Model file for the job. Use its own axes, mm. Round coordinates to 2 decimals unless told otherwise and drop trailing zeros. Order: outer loops, then holes, each group sorted by start corner. A loop starts at its lowest first (then second) coordinate and runs counter-clockwise, first axis right, second up. Notation, with made-up numbers: (64.5, 5.5) -> (79.5, 5.5) arc R15 cw to (79.5, 31.5) -> close; hole circle Ø5 at (-38, 57.5). An arc over 180 degrees is marked (long way). Answer as CSV lines item,"result".
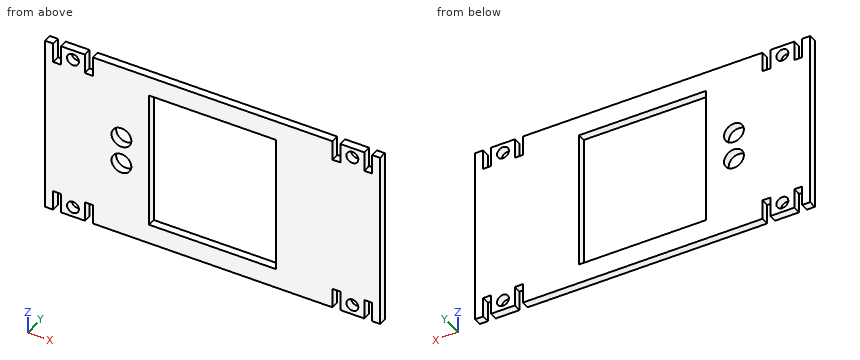
```python
from build123d import *

# Parameters (mm, degrees)
SKETCH1_R           = 1.5
BOSS_EXTRUDE1_DEPTH = 2
SKETCH2_W           = 32
SKETCH2_H           = 35
CUT_EXTRUDE1_DEPTH  = 10
SKETCH3_R           = 2.5
CUT_EXTRUDE2_DEPTH  = 10


with BuildPart() as part:
    # Sketch1 → Boss-Extrude1 (new body)
    with BuildSketch(Plane(origin=(0, 0, 0), x_dir=(1, 0, 0), z_dir=(0, 1, 0))):
        Polygon((0, 0), (2, 0), (2, 5), (4, 5), (4, 0), (10, 0), (10, 5), (12, 5), (12, 0), (72.4, 0), (72.4, 5), (74.4, 5), (74.4, 0), (80.4, 0), (80.4, 5), (82.4, 5), (82.4, 0), (84.4, 0), (84.4, 45), (82.4, 45), (82.4, 40), (80.4, 40), (80.4, 45), (74.4, 45), (74.4, 40), (72.4, 40), (72.4, 45), (12, 45), (12, 40), (10, 40), (10, 45), (4, 45), (4, 40), (2, 40), (2, 45), (0, 45), align=None)
        with Locations(Location((7, 42.5, 0), (0, 0, 270))):
            Circle(SKETCH1_R, mode=Mode.SUBTRACT)
        with Locations(Location((77.4, 42.5, 0), (0, 0, 90))):
            Circle(SKETCH1_R, mode=Mode.SUBTRACT)
        with Locations(Location((7, 2.5, 0), (0, 0, 90))):
            Circle(SKETCH1_R, mode=Mode.SUBTRACT)
        with Locations(Location((77.4, 2.5, 0), (0, 0, 270))):
            Circle(SKETCH1_R, mode=Mode.SUBTRACT)
    extrude(amount=BOSS_EXTRUDE1_DEPTH)

    # Sketch2 → Cut-Extrude1 (cut)
    with BuildSketch(Plane(origin=(0, 2, 0), x_dir=(1, 0, 0), z_dir=(0, 1, 0))):
        with Locations((42.2, 22.5)):
            Rectangle(SKETCH2_W, SKETCH2_H)
    extrude(amount=-CUT_EXTRUDE1_DEPTH, mode=Mode.SUBTRACT)

    # Sketch3 → Cut-Extrude2 (cut)
    with BuildSketch(Plane(origin=(0, 2, 0), x_dir=(1, 0, 0), z_dir=(0, 1, 0))):
        with Locations(Location((19.2, 26, 0), (0, 0, 270))):
            Circle(SKETCH3_R)
        with Locations(Location((19.2, 19, 0), (0, 0, 90))):
            Circle(SKETCH3_R)
    extrude(amount=-CUT_EXTRUDE2_DEPTH, mode=Mode.SUBTRACT)


solid = part.part
```
Q1. Saw through at C-C (x = 36). Write the cut outline in (y, z).
Checks:
outline,"(0, -45) -> (2, -45) -> (2, -40) -> (0, -40) -> close; (0, -5) -> (2, -5) -> (2, 0) -> (0, 0) -> close"
Q2. Saw through at B-B (z = -32). Write the cut outline in (x, y), plus the area to 3 significant figures.
Checks:
outline,"(0, 0) -> (26.2, 0) -> (26.2, 2) -> (0, 2) -> close; (58.2, 0) -> (84.4, 0) -> (84.4, 2) -> (58.2, 2) -> close"
area,"105 mm²"
Q3. Saw through at D-D (z = -2.5). Write the cut outline in (x, y).
Checks:
outline,"(0, 0) -> (2, 0) -> (2, 2) -> (0, 2) -> close; (4, 0) -> (5.5, 0) -> (5.5, 2) -> (4, 2) -> close; (8.5, 0) -> (10, 0) -> (10, 2) -> (8.5, 2) -> close; (12, 0) -> (72.4, 0) -> (72.4, 2) -> (12, 2) -> close; (74.4, 0) -> (75.9, 0) -> (75.9, 2) -> (74.4, 2) -> close; (78.9, 0) -> (80.4, 0) -> (80.4, 2) -> (78.9, 2) -> close; (82.4, 0) -> (84.4, 0) -> (84.4, 2) -> (82.4, 2) -> close"
Q4. Saw through at A-A (x = 19.2). Write the cut outline in (y, z).
Checks:
outline,"(0, -45) -> (2, -45) -> (2, -28.5) -> (0, -28.5) -> close; (0, -23.5) -> (2, -23.5) -> (2, -21.5) -> (0, -21.5) -> close; (0, -16.5) -> (2, -16.5) -> (2, 0) -> (0, 0) -> close"
Q5. Wall check: L1, parallel to Z at x = 77.4, y = 1.55; L2, parallel to X at y = 1.35, z = -19; L3, parallel to Z at x = 41, y = 1.3. Give the ranges that are in metal, low to high. Write a range as [from, to].
Checks:
L1,"[-45, -44], [-41, -4], [-1, 0]"
L2,"[0, 16.7], [21.7, 26.2], [58.2, 84.4]"
L3,"[-45, -40], [-5, 0]"
Q6. Flat gauge pins, fed straight in: pin 1 (2 mm diameter, centred on x = 60, z = -39, fed in from -Y); pin 2 (0.6 mm diameter, centred on x = 3, y = 0.5, fed in from +Z). Where does each tip first touch, or does it go through?
Checks:
pin 1,"y = 0"
pin 2,"z = -5"
